Part model, mm, in its own coordinate system. A direction names the side the tool comes from. Coordinates: 2 decimals unless noted, no trailing zeros. Write each loop counter-clockwise with the first axis right and the second up, starting at its lowest first coordinate (ties: lowest second). Pieces come first, ordered by that corner, then holes. Notation, with made-up numbers: (-25, 76) - (-4, 76) arc R24 cw to (-4, 112) - close; hole circle Ø8 at (-21, 31.5). An arc over 180 degrees is marked (long way). Use a Markdown table: item, result.
Autodesk Inventor part; units mm, degrees
ref_plane "YZ Plane" through (0, 0, 0) normal (1, 0, 0) x (0, 1, 0)
ref_plane "XZ Plane" through (0, 0, 0) normal (0, 1, 0) x (-1, 0, 0)
ref_plane "XY Plane" through (0, 0, 0) normal (0, 0, 1) x (1, 0, 0)
sketch "Sketch1" plane through (0, 0, 0) normal (0, 0, 1) x (1, 0, 0)
  line L0 (0, 0) -> (62, 30) construction
  line L1 (62, 30) -> (70, 30) construction
  line L2 (20.2572, 9.8019) -> (25, 0) construction
  circle A0 centre (0, 0) radius 1.5
  circle A1 centre (25, 0) radius 1
  arc A2 (2.5837, 2.3611) -> (3.4548, 0.5608) centre (0, 0) ccw
  arc A3 (23.7065, 1.5254) -> (24.6066, 1.9609) centre (25, 0) ccw
  line L3 (3.4548, 0.5608) -> (20.2426, 8.6839)
  line L4 (20.2426, 8.6839) -> (23.7065, 1.5254)
  line L5 (24.6066, 1.9609) -> (21.1428, 9.1195)
  line L6 (21.1428, 9.1195) -> (62.2292, 29)
  line L7 (62.2292, 29) -> (70, 29)
  arc A4 (70, 29) -> (70, 31) centre (70, 30) ccw
  line L8 (70, 31) -> (61.7708, 31)
  line L9 (61.7708, 31) -> (2.5837, 2.3611)
  dimension "d0" = 25
  dimension "d1" = 70
  dimension "d2" = 8
  dimension "d3" = 30
  dimension "d4" = 3
  dimension "d5" = 2
  dimension "d6" = 7
  dimension "d7" = 4
  dimension "d8" = 1
  dimension "d9" = 1
  dimension "d10" = 1
  dimension "d11" = 1
  dimension "d12" = 0.5
  dimension "d13" = 0.5
extrude "Extrusion1" add sketch "Sketch1" along normal mid plane 10
fillet "Fillet1" radius 2 8 edges at (3.4548, 0.5608, 0) (2.5837, 2.3611, 0) (21.1428, 9.1195, 0) (20.2426, 8.6839, 0) (62.2292, 29, 0) (61.7708, 31, 0) (24.6066, 1.9609, 0) (23.7065, 1.5254, 0)
properties material "Aluminum 6061"
Item 1: Which spindle directions (+Z, -Z, +X, -X, +Y, -Y) get a long thin tool onto all of the face, cutting with end or side? Do faces 4 (the face through (66, 29, 0)), 5 (the face through (3.84, 0.486, 0.07)), 6 (the face through (28, 14, -5)). Say none if no direction does.
From the geometry:
| item | result |
|---|---|
| face 4 | +Z, -Z, +X, -Y |
| face 5 | +Z, -Z, -Y |
| face 6 | -Z, +X, -X, +Y, -Y |
Item 2: Band-saw the part on A-A, the plane x = 0. Give the cut face in (y, z), then the cut area to 3 significant figures.
From the geometry:
| item | result |
|---|---|
| outline | (-3.5, -5) - (-1.5, -5) - (-1.5, 5) - (-3.5, 5) - close; (1.5, -5) - (3.5, -5) - (3.5, 5) - (1.5, 5) - close |
| area | 40.0 mm^2 |
Item 3: Drill centre lines: probe 1 along Y at (x, z) = (0, 0.75); probe 2 along Y at (x, z) = (25, -1.25); probe 3 along X at (y, z) = (-0.5, 1). Where is each one in solid material? Low to high.
From the geometry:
| item | result |
|---|---|
| probe 1 | -3.5 to -1.5, 1.5 to 3.5 |
| probe 2 | -2 to -1, 1 to 2.11, 10.99 to 13.21 |
| probe 3 | -3.46 to -1.41, 1.41 to 3.46, 23.06 to 24.13, 25.87 to 26.94 |
Item 4: Band-saw the part on B-B, the plane z = -3.25. Give the cut face in (x, y).
From the geometry:
| item | result |
|---|---|
| outline | (1.81, 3) arc R3.5 ccw (long way) to (3.47, -0.44) arc R2 cw to (4.59, 1.11) - (18.44, 7.81) arc R2 cw to (21.11, 6.88) - (23.19, 2.59) arc R2 cw to (23.19, 0.86) arc R2 ccw (long way) to (25.45, 1.95) arc R2 cw to (24.09, 3.03) - (22.01, 7.32) arc R2 cw to (22.94, 9.99) - (61.82, 28.8) arc R2 cw to (62.69, 29) - (70, 29) arc R1 ccw to (70, 31) - (62.23, 31) arc R2 ccw to (61.36, 30.8) - (3.71, 2.91) arc R2 cw to start; hole circle Ø3 at (0, 0); hole circle Ø2 at (25, 0) |
Item 5: Two-plate mould, pull along X, no slides. Class faces 1 (the face through (22.137, 4.768, -0.07)), 2 (the face through (23.07, 5.14, -0.07)), 3 (the face through (66, 31, 0)): pulls with the +X half, pulls with the -X half, needs draft (parallel to the pull), parting line crosses it, or undercut.
From the geometry:
| item | result |
|---|---|
| face 1 | undercut |
| face 2 | pulls with the +X half |
| face 3 | needs draft |
Item 6: Drop flat-ended pins along their axis: P1, Ø4, axis at x = 34.5, y = 15.5, coming from the +Z side; P2, Ø3, axis at x = 15, z = 1.5, coming from the +Y side; P3, Ø1, axis at y = 21, z = 0.5, coming from the +X side; P4, Ø6, axis at x = 67.5, z = 1.5, coming from the -Y side. Give the stop position or say it passes through.
From the geometry:
| item | result |
|---|---|
| P1 | z = 5 |
| P2 | y = 9.09 |
| P3 | x = 46.73 |
| P4 | y = 29 |
Item 7: Band-saw the part on C-C, the plane y = 30. Give the cut face in (x, z).
From the geometry:
| item | result |
|---|---|
| outline | (59.7, -5) - (71, -5) - (71, 5) - (59.7, 5) - close |
Item 8: Band-saw the part on D-D, the plane x = 45. Give the cut face in (y, z).
From the geometry:
| item | result |
|---|---|
| outline | (20.66, -5) - (22.89, -5) - (22.89, 5) - (20.66, 5) - close |
